Geometry: see drawing. Coordinates: mm, zero at the bounding-box minimum. Coordinates: 2 decimals unless noted, no trailing zeros. Write each loop counter-clockwise with the first axis right and the second up, starting at its lowest first coordinate (ties: lowest second). Pieces come first, ordered by that corner, then holes. Notation, with made-up numbers: M 40.25,-4.5 L 92.25,-4.5 A28 cw 92.25,28.5 Z; hole C -18,51.25 d3. An arc over 180 degrees is marked long. One line per item, written item: value. Start each with the question number.
Item 1: Cut plane C-C, the plane z = 0.3. Output: boundary loops of the cut face in (x, y).
Item 2: Cut plane B-B, the plane y = 35. Output: boundary loops of the cut face in (x, z).
Item 3: Cut plane A-A, the plane x = 15.5. Output: boundary loops of the cut face in (y, z), then the cut area to 3 significant figures.
Item 4: Cut plane D-D, the plane y = 63. Output: boundary loops of the cut face in (x, z).
Item 5: Ray query, L1, parallel to X at y = 6, z = 0.65 (1 decimal); L2, parallel to X at y = 7.5, z = 0.3 (1 decimal); L3, parallel to Y at x = 15, z = 0.3. Return the intervals inside material, ascending. Write a range as from..to.
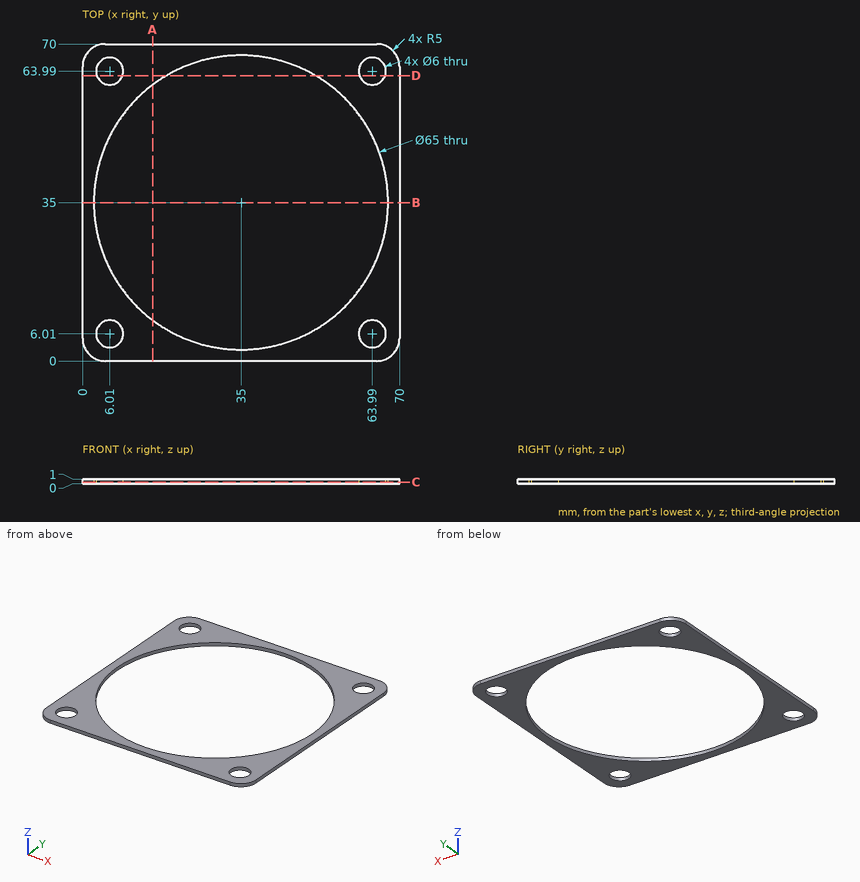
From the geometry:
1. outline: M 0,5 A5 ccw 5,0 L 65,0 A5 ccw 70,5 L 70,65 A5 ccw 65,70 L 5,70 A5 ccw 0,65 Z; hole C 35,35 d65; hole C 6.01,6.01 d6; hole C 6.01,63.99 d6; hole C 63.99,6.01 d6; hole C 63.99,63.99 d6
2. outline: M 0,0 L 2.5,0 L 2.5,1 L 0,1 Z; M 67.5,0 L 70,0 L 70,1 L 67.5,1 Z
3. outline: M 0,0 L 9,0 L 9,1 L 0,1 Z; M 61,0 L 70,0 L 70,1 L 61,1 Z
3. area: 18.0 mm²
4. outline: M 0,0 L 3.18,0 L 3.18,1 L 0,1 Z; M 8.84,0 L 18.5,0 L 18.5,1 L 8.84,1 Z; M 51.5,0 L 61.16,0 L 61.16,1 L 51.5,1 Z; M 66.82,0 L 70,0 L 70,1 L 66.82,1 Z
5. L1: x = 0..3, 9..20.3, 49.7..61, 67..70
5. L2: x = 0..3.4, 8.6..17.7, 52.3..61.4, 66.6..70
5. L3: y = 0..9.38, 60.62..70
